```python
from build123d import *

# Parameters (mm, degrees)
F1_DEPTH             = 18
F4_D                 = 4.4
F4_CBORE_D           = 8.25
F4_CBORE_DEPTH       = 4
F4_ON_F3_D           = 4.4
F4_ON_F3_CBORE_D     = 8.25
F4_ON_F3_CBORE_DEPTH = 4
F5_SIZE              = 2
F6_R                 = 1
F7_R                 = 1.65
F8_DEPTH             = 15.001
F9_R                 = 4
F10_DEPTH            = 3


with BuildPart() as f1:
    # F0 (on Top) → F1 (new body)
    with BuildSketch(Plane.XY):
        Polygon((0, 6), (0, 0), (16, 0), (16, 10), (42, 10), (42, 0), (58, 0), (58, 6), (46, 6), (46, 15), (42.25, 18.75), (42.25, 43), (38.25, 43), (38.25, 15), (19.75, 15), (19.75, 43), (15.75, 43), (15.75, 18.75), (12, 15), (12, 6), align=None)
    extrude(amount=F1_DEPTH)

    # F4 (through all)
    with Locations(Plane(origin=(0, 6, 0), x_dir=(-1, 0, 0), z_dir=(0, 1, 0))):
        with Locations((-52, 9)):
            CounterBoreHole(F4_D / 2, F4_CBORE_D / 2, F4_CBORE_DEPTH)

    # F4 on F3 (through all)
    with Locations(Plane(origin=(0, 6, 0), x_dir=(-1, 0, 0), z_dir=(0, 1, 0))):
        with Locations((-6, 9)):
            CounterBoreHole(F4_ON_F3_D / 2, F4_ON_F3_CBORE_D / 2, F4_ON_F3_CBORE_DEPTH)

    # F5
    f5_edges = [f1.edges().sort_by_distance(p)[0] for p in [
        (16, 10, 9),
        (42, 10, 9),
    ]]
    chamfer(f5_edges, length=F5_SIZE)

    # F6
    f6_edges = [f1.edges().sort_by_distance(p)[0] for p in [
        (46, 6, 9),
        (38.25, 43, 9),
        (19.75, 43, 9),
        (12, 6, 9),
        (0, 6, 9),
        (58, 6, 9),
        (12, 15, 9),
        (15.75, 43, 9),
        (46, 15, 9),
        (42.25, 43, 9),
    ]]
    fillet(f6_edges, radius=F6_R)

    # F7 (on face) → F8 (cut, through all)
    with BuildSketch(Plane(origin=(0, 15, 0), x_dir=(-1, 0, 0), z_dir=(0, 1, 0))):
        with Locations((-29, 9)):
            Circle(F7_R)
    extrude(amount=-F8_DEPTH, mode=Mode.SUBTRACT)

    # F9 (on face) → F10 (cut)
    with BuildSketch(Plane(origin=(0, 15, 0), x_dir=(-1, 0, 0), z_dir=(0, 1, 0))):
        with Locations((-29, 9)):
            Circle(F9_R)
    extrude(amount=-F10_DEPTH, mode=Mode.SUBTRACT)


solid = f1.part
```
Part model, mm, in its own coordinate system. A direction names the side the tool comes from. Round coordinates to 2 decimals unless told otherwise and drop trailing zeros. Order: outer loops, then holes, each group sorted by start corner. A loop starts at its lowest first (then second) coordinate and runs counter-clockwise, first axis right, second up. Notation, with made-up numbers: M 70.5,-11.75 L 88.5,-11.75 A13 cw 88.5,3.25 Z; hole C -27,-38 d7. An arc over 180 degrees is marked long. Answer in a Markdown table with one row per item. Add a question column.
Q1. Cut at A-A on x = 29. Give the cut face in (y, z), and give its area (3 significant figures).
Q2. Cut at C-C on z = 9. Give the number of separate pieces and of enclosed holes in the cut face, and give its area (3 significant figures).
Q3. Pin check, flat tips, straight feed: pin 1 (3 mm diameter, centred on x = 18, y = 38.5, fed in from -Z); pin 2 (4 mm diameter, centred on y = 12, z = 5.5, fed in from +X); pin 3 (9 mm diameter, centred on x = 30, z = 13, fed in from +Y); pin 4 (2.5 mm diameter, centred on x = 51.5, z = 10, fed in from +Y). Stop position of each tip, or through.
Q4. 3-axis set-ups, long thin cutter, end or side, ignore diameter. For faces 1 (the face through (17, 9, 9)), 2 (the face through (55.273, 4.028, 6.49)), 3 (the face through (38.25, 29, 9)), 4 (the face through (12, 11, 9)): which of +Z, -Z, +X, -X, +Y, -Y reach the whole face in a straight line?
Q5. Cut at D-D on y = 11. Give the cut face in (x, z).
Q6. Wall check: L1, parallel to X at y = 32, z = 6.5; L2, parallel to X at y = 5, z = 11; L3, parallel to Z at x = 6, y = 5.1 (3 decimals). Give the ranges that are in metal, low to high. Write a range as from..to.
Q7. Cut at B-B on y = 32. Give the cut face in (x, z).
Q8. Mould opens along X. For faces 5 (the face through (40, 43, 9)), 6 (the face through (42, 4, 9)), 7 (the face through (42.25, 30, 9)) say: +X half, -X half, draft (parallel to the pull), parting line (faces both ways), or undercut.
Established:
| question | item | result |
|---|---|---|
| 1 | outline | M 10,0 L 15,0 L 15,5 L 12,5 L 12,7.35 L 10,7.35 Z; M 10,10.65 L 12,10.65 L 12,13 L 15,13 L 15,18 L 10,18 Z |
| 1 | area | 59.4 mm2 |
| 2 | separate pieces | 4 |
| 2 | enclosed holes | 0 |
| 2 | area | 521 mm2 |
| 3 | pin 1 | stops at z = 0 |
| 3 | pin 2 | stops at x = 46 |
| 3 | pin 3 | stops at y = 15 |
| 3 | pin 4 | stops at y = 2 |
| 4 | face 1 | +Z, -Z, -Y |
| 4 | face 2 | +Y |
| 4 | face 3 | +Z, -Z, +Y |
| 4 | face 4 | +Z, -Z, -X, +Y |
| 5 | outline | M 12,0 L 46,0 L 46,18 L 12,18 Z; hole C 29,9 d3.3 |
| 6 | L1 | x = 15.75..19.75, 38.25..42.25 |
| 6 | L2 | x = 0..2.39, 9.61..16, 42..48.39, 55.61..58 |
| 6 | L3 | z = 0..4.875, 13.125..18 |
| 7 | outline | M 15.75,0 L 19.75,0 L 19.75,18 L 15.75,18 Z; M 38.25,0 L 42.25,0 L 42.25,18 L 38.25,18 Z |
| 8 | face 5 | draft |
| 8 | face 6 | undercut |
| 8 | face 7 | +X half |
